Can you work these out from the drawing? Everything is in mm from the part's minimum corner. A direction names the side the tool comes from. Round coordinates to 2 decimals unless told otherwise and drop trailing zeros. Loops run counter-clockwise (first coordinate to the right, second up) from the corner with the lowest first, then second, coordinate; pieces in that order, holes last. Notation, with made-up numbers: (17.5, 82) -> (31.5, 82) arc R11 cw to (31.5, 86) -> close; hole circle Ø1 at (18.5, 56). An arc over 180 degrees is marked (long way). Answer as a JSON object with one key per item and string values.
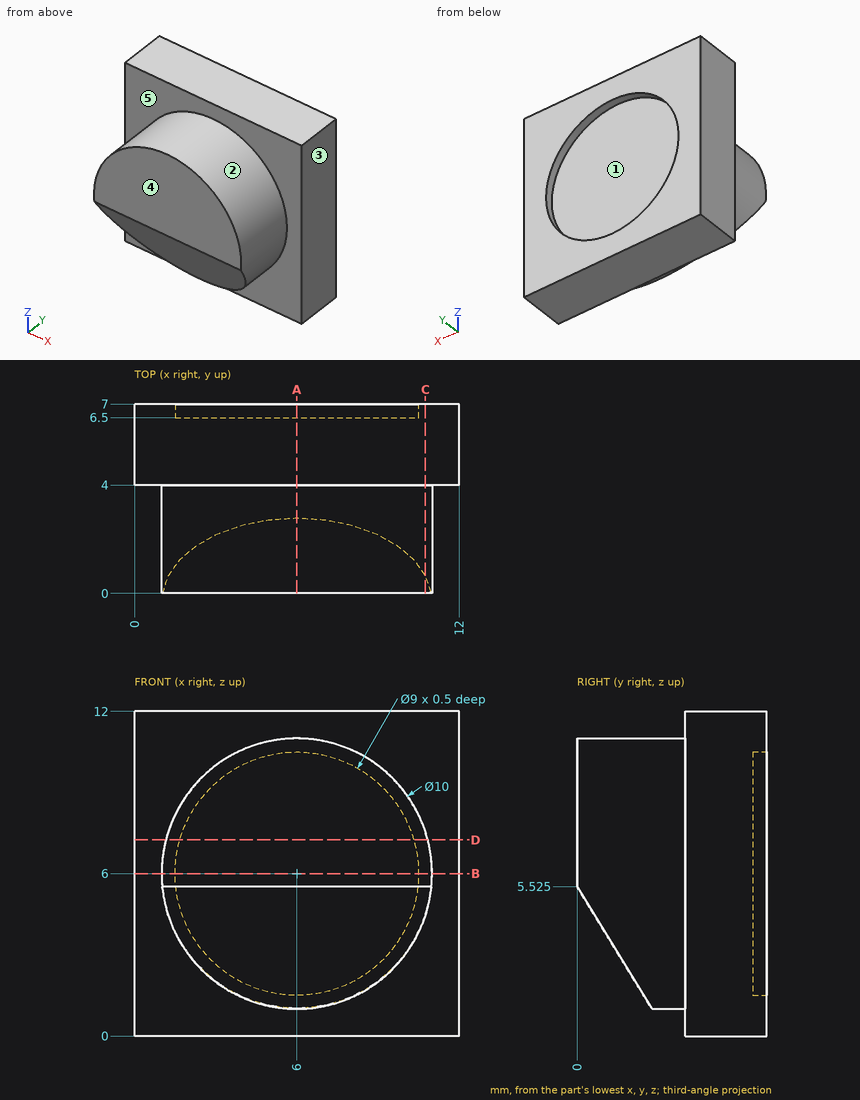
Q1. I want a section at A-A, the plane x = 6. Write out the boundary of the cut face in (y, z) (1 decimal).
Determined:
{"outline": "(0, 5.5) -> (2.8, 1) -> (4, 1) -> (4, 0) -> (7, 0) -> (7, 1.5) -> (6.5, 1.5) -> (6.5, 10.5) -> (7, 10.5) -> (7, 12) -> (4, 12) -> (4, 11) -> (0, 11) -> close"}
Q2. On a 3-axis mill with a long thin cutter (end or side, diameter ignored), from which of +Z, -Z, +X, -X, +Y, -Y can I reach the whole of each face in a straight line? I mean the marked faces 4 and 5. Say none if no direction works.
Determined:
{"face 4": "+Z, -Z, +X, -X, -Y", "face 5": "-Y"}
Q3. I want a section at B-B, the plane z = 6. Write out the boundary of the cut face in (x, y).
Determined:
{"outline": "(0, 4) -> (1, 4) -> (1, 0) -> (11, 0) -> (11, 4) -> (12, 4) -> (12, 7) -> (10.5, 7) -> (10.5, 6.5) -> (1.5, 6.5) -> (1.5, 7) -> (0, 7) -> close"}
Q4. If I drill on L1, parallel to Z at x = 6, y = 6.75; L2, parallel to X at y = 6.75, z = 7; L3, parallel to Y at x = 6.75, z = 6.25, over which ranges is the centre line in solid material (lowest first)? Write a range as [from, to].
Determined:
{"L1": "[0, 1.5], [10.5, 12]", "L2": "[0, 1.61], [10.39, 12]", "L3": "[0, 6.5]"}
Q5. I want a section at C-C, the plane x = 10.75. Write out the boundary of the cut face in (y, z) (1 decimal).
Determined:
{"outline": "(0, 5.5) -> (0.7, 4.4) -> (4, 4.4) -> (4, 0) -> (7, 0) -> (7, 12) -> (4, 12) -> (4, 7.6) -> (0, 7.6) -> close"}
Q6. We'd pull the mould along Z, two halves only. Please class the marked faces 1, 2 and 3: pulls with the +Z half, pulls with the -Z half, needs draft (parallel to the pull), parting line crosses it, or undercut.
Determined:
{"face 1": "undercut", "face 2": "parting line crosses it", "face 3": "needs draft"}
Q7. I want a section at D-D, the plane z = 7.25. Write out the boundary of the cut face in (x, y).
Determined:
{"outline": "(0, 4) -> (1.16, 4) -> (1.16, 0) -> (10.84, 0) -> (10.84, 4) -> (12, 4) -> (12, 7) -> (10.32, 7) -> (10.32, 6.5) -> (1.68, 6.5) -> (1.68, 7) -> (0, 7) -> close"}
Q8. I'm going to push flat-ended pins straight in: pin 1 (4 mm diameter, centred on x = 2.5, z = 2.5, fed in from -Y); pin 2 (4.5 mm diameter, centred on x = 6, z = 7, fed in from +Y). Where does each tip first touch, or does it pass through?
Determined:
{"pin 1": "y = 0.63", "pin 2": "y = 6.5"}
